from build123d import *

# Parameters (mm, degrees)
BOSS_EXTRUDE1_DEPTH = 5
FILLET1_R           = 5
CHAMFER1_SIZE       = 8
FILLET2_R           = 4
SKETCH2_R           = 2.1
CUT_EXTRUDE1_DEPTH  = 271.24803422
SKETCH3_R           = 3.9
CUT_EXTRUDE2_DEPTH  = 3
BOSS_EXTRUDE2_START = 1
SKETCH4_R           = 5.4
SKETCH4_R_2         = 3.9
BOSS_EXTRUDE2_DEPTH = 1
FILLET3_R           = 3


with BuildPart() as part:
    # Sketch1 → Boss-Extrude1 (new body)
    with BuildSketch(Plane.XY):
        Polygon((-255, 28), (-255, -2), (-234, -2), (-226, -10), (-178, -10), (-170, -2), (-170, 23), (-207, 23), (-210, 28), align=None)
    boss_extrude1 = extrude(amount=BOSS_EXTRUDE1_DEPTH)

    # Mirror1: Boss-Extrude1 across plane
    add(boss_extrude1.mirror(Plane(origin=(-125, 0, -125), x_dir=(-0.7071067811865489, 0, 0.7071067811865462), z_dir=(-0.7071067811865464, 0, -0.7071067811865488))))

    # Fillet1
    fillet1_edges = [part.edges().sort_by_distance(p)[0] for p in [
        (-210, 28, 2.5),
        (-207, 23, 2.5),
        (-170, 23, 2.5),
        (-170, -2, 2.5),
        (-178, -10, 2.5),
        (-226, -10, 2.5),
        (-234, -2, 2.5),
        (-252.5, -2, -16),
        (-252.5, 28, -40),
        (-252.5, 23, -43),
        (-252.5, 23, -80),
        (-252.5, -2, -80),
        (-252.5, -10, -72),
        (-252.5, -10, -24),
    ]]
    fillet(fillet1_edges, radius=FILLET1_R)

    # Chamfer1
    chamfer1_edges = [part.edges().sort_by_distance(p)[0] for p in [
        (-255, 13, 5),
    ]]
    chamfer(chamfer1_edges, length=CHAMFER1_SIZE)

    # Fillet2
    fillet2_edges = [part.edges().sort_by_distance(p)[0] for p in [
        (-247, 13, 5),
        (-255, 13, -3),
    ]]
    fillet(fillet2_edges, radius=FILLET2_R)

    # Sketch2 → Cut-Extrude1 (cut, through all)
    with BuildSketch(Plane.XY.offset(5)):
        with Locations((-218, 3.425126266)):
            Circle(SKETCH2_R)
        with Locations((-186, 3.425126266)):
            Circle(SKETCH2_R)
    cut_extrude1 = extrude(amount=-CUT_EXTRUDE1_DEPTH, mode=Mode.SUBTRACT)

    # Sketch3 → Cut-Extrude2 (cut)
    with BuildSketch(Plane.XY.offset(5)):
        with Locations((-218, 3.425126266)):
            Circle(SKETCH3_R)
        with Locations((-186, 3.425126266)):
            Circle(SKETCH3_R)
    cut_extrude2 = extrude(amount=-CUT_EXTRUDE2_DEPTH, mode=Mode.SUBTRACT)

    # Sketch4 → Boss-Extrude2 (add)
    # profile 1 of 2: a face of its own
    with BuildSketch(Plane.XY.offset(5).offset(BOSS_EXTRUDE2_START)):
        with Locations((-218, 3.425126266)):
            Circle(SKETCH4_R)
        with Locations((-218, 3.425126266)):
            Circle(SKETCH4_R_2, mode=Mode.SUBTRACT)
    # profile 2 of 2: a face of its own
    with BuildSketch(Plane.XY.offset(5).offset(BOSS_EXTRUDE2_START)):
        with Locations((-186, 3.425126266)):
            Circle(SKETCH4_R)
        with Locations((-186, 3.425126266)):
            Circle(SKETCH4_R_2, mode=Mode.SUBTRACT)
    boss_extrude2 = extrude(amount=-BOSS_EXTRUDE2_DEPTH)

    # Mirror2: Cut-Extrude1, Cut-Extrude2, Boss-Extrude2 across plane
    add(cut_extrude1.mirror(Plane(origin=(-125, 0, -125), x_dir=(-0.7071067811865489, 0, 0.7071067811865462), z_dir=(-0.7071067811865464, 0, -0.7071067811865488))), mode=Mode.SUBTRACT)
    add(cut_extrude2.mirror(Plane(origin=(-125, 0, -125), x_dir=(-0.7071067811865489, 0, 0.7071067811865462), z_dir=(-0.7071067811865464, 0, -0.7071067811865488))), mode=Mode.SUBTRACT)
    add(boss_extrude2.mirror(Plane(origin=(-125, 0, -125), x_dir=(-0.7071067811865489, 0, 0.7071067811865462), z_dir=(-0.7071067811865464, 0, -0.7071067811865488))))

    # Fillet3
    # the kernel refuses this fillet: 3 mm, written as the material it adds along each edge
    with BuildSketch(Plane(origin=(-218, 3.425126266, 5), x_dir=(1, 0, 0), z_dir=(0, -1, 0))) as fillet3_piece_1:
        with BuildLine():
            CenterArc((7.636067977, 3), FILLET3_R, 221.810314896, 48.189685104)
            Line((5.4, 1), (5.35527864, 0.96))
            ThreePointArc((5.35527864, 0.96), (5.34, 0.5), (5.34, 0))
            Line((5.34, 0), (5.4, -0.06))
            Line((5.4, -0.06), (7.636067977, -0.06))
            Line((7.636067977, -0.06), (7.636067977, 0))
        make_face()
    revolve(axis=Axis((-218, 3.425126266, 5), (0, 0, 1)))
    with BuildSketch(Plane(origin=(-186, 3.425126266, 5), x_dir=(1, 0, 0), z_dir=(0, -1, 0))) as fillet3_piece_2:
        with BuildLine():
            CenterArc((7.636067977, 3), FILLET3_R, 221.810314896, 48.189685104)
            Line((7.636067977, 0), (7.636067977, -0.06))
            Line((7.636067977, -0.06), (5.4, -0.06))
            Line((5.4, -0.06), (5.34, 0))
            ThreePointArc((5.34, 0), (5.34, 0.5), (5.35527864, 0.96))
            Line((5.35527864, 0.96), (5.4, 1))
        make_face()
    revolve(axis=Axis((-186, 3.425126266, 5), (0, 0, 1)))
    with BuildSketch(Plane(origin=(-255, 3.425126266, -32), x_dir=(0, 0, -1), z_dir=(0, -1, 0))) as fillet3_piece_3:
        with BuildLine():
            CenterArc((7.636067977, -3), FILLET3_R, 90, 48.189685104)
            Line((5.4, -1), (5.35527864, -0.96))
            ThreePointArc((5.35527864, -0.96), (5.34, -0.5), (5.34, 0))
            Line((5.34, 0), (5.4, 0.06))
            Line((5.4, 0.06), (7.636067977, 0.06))
            Line((7.636067977, 0.06), (7.636067977, 0))
        make_face()
    revolve(axis=Axis((-255, 3.425126266, -32), (1, 0, 0)))
    with BuildSketch(Plane(origin=(-255, 3.425126266, -64), x_dir=(0, 0, -1), z_dir=(0, -1, 0))) as fillet3_piece_4:
        with BuildLine():
            CenterArc((7.636067977, -3), FILLET3_R, 90, 48.189685104)
            Line((5.4, -1), (5.35527864, -0.96))
            ThreePointArc((5.35527864, -0.96), (5.34, -0.5), (5.34, 0))
            Line((5.34, 0), (5.4, 0.06))
            Line((5.4, 0.06), (7.636067977, 0.06))
            Line((7.636067977, 0.06), (7.636067977, 0))
        make_face()
    revolve(axis=Axis((-255, 3.425126266, -64), (1, 0, 0)))


solid = part.part
Read the model definition and answer for the solid it produces. Units are mm, in the model's axes. A direction names the side the tool comes from. Coordinates: 2 decimals unless noted, no trailing zeros. Write each loop counter-clockwise with the first axis right and the second up, starting at its lowest first coordinate (ties: lowest second). Pieces come first, ordered by that corner, then holes. Notation, with made-up numbers: M -8,-28.5 L 41,-28.5 A17 ccw 41,-22.5 Z; hole C 89.25,84 d7. An arc over 180 degrees is marked long. Use a Markdown table: item, result.
Q1. The part is cut by section B-B, the plane x = -186. Write down the section's boundary in (y, z), then the cut area to 3 significant figures.
Answer block:
| item | result |
|---|---|
| outline | M -10,0 L 1.33,0 L 1.33,2 L -0.47,2 L -0.47,6 L -1.97,6 A3 cw -4.21,5 L -10,5 Z; M 5.53,0 L 23,0 L 23,5 L 11.06,5 A3 cw 8.83,6 L 7.33,6 L 7.33,2 L 5.53,2 Z |
| area | 138 mm2 |
Q2. Each of these flat-tipped pins is pushed along its axis until it touches: pin 1 Ø19 at (x, y) = (-189.5, 18.5) entering from +Z; pin 2 Ø4 at (x, y) = (-184.5, 2.5) entering from +Z; pin 3 Ø2 at (y, z) = (8.5, -48) entering from -X. Where does it stop, or does it pass through?
Answer block:
| item | result |
|---|---|
| pin 1 | stops at z = 5.5 |
| pin 2 | stops at z = 2 |
| pin 3 | stops at x = -255 |
Q3. Straight lines are drawn through the part: L1, parallel to Y at x = -186, z = 4.5; L2, parallel to Y at x = -218, z = 2.8; L3, parallel to X at y = 20, z = -44. For each, find the intervals that lie inside material, in ascending order. Write a range as [from, to].
Answer block:
| item | result |
|---|---|
| L1 | y = [-10, -0.47], [7.33, 23] |
| L2 | y = [-10, -0.47], [7.33, 28] |
| L3 | x = [-255, -250] |
Q4. Which of the six approach directions +Z, -Z, +X, -X, +Y, -Y give full straight-line access (tool end or side, diameter ignored) to faces 4 (the face through (-250, 9, -39)), 5 (the face through (-189, 23, 2)), 6 (the face through (-252, 2, -34))?
Answer block:
| item | result |
|---|---|
| face 4 | -Z, +X, +Y, -Y |
| face 5 | +Z, -Z, +X, +Y |
| face 6 | -X |
Q5. Determine the mould class of faces 1 (the face through (-211, 9, 0)), 2 (the face through (-189.896, 3.597, 4.028)), 3 (the face through (-206.6, 23.63, 2.54)) for opening direction X: released by +X, released by -X, zero draft, split by the parting line, or undercut.
Answer block:
| item | result |
|---|---|
| face 1 | zero draft |
| face 2 | undercut |
| face 3 | released by +X |
Q6. The part is cut by section D-D, the plane z = -44. Write down the section's boundary in (x, y), then the cut area to 3 significant figures.
Answer block:
| item | result |
|---|---|
| outline | M -255,-10 L -250,-10 L -250,23.35 L -255,23.35 Z |
| area | 167 mm2 |
Q7. The part is cut by section A-A, the plane z = -32. Write down the section's boundary in (x, y).
Answer block:
| item | result |
|---|---|
| outline | M -256,-1.97 A3 cw -255,-4.21 L -255,-10 L -250,-10 L -250,1.33 L -252,1.33 L -252,-0.47 L -256,-0.47 Z; M -256,7.33 L -252,7.33 L -252,5.53 L -250,5.53 L -250,28 L -255,28 L -255,11.06 A3 cw -256,8.83 Z |
Q8. The part is cut by section C-C, the plane y = -6.5. Write down the section's boundary in (x, z).
Answer block:
| item | result |
|---|---|
| outline | M -255,-75.5 L -250,-75.5 L -250,-20.5 L -255,-20.5 Z; M -229.5,0 L -174.5,0 L -174.5,5 L -229.5,5 Z |
